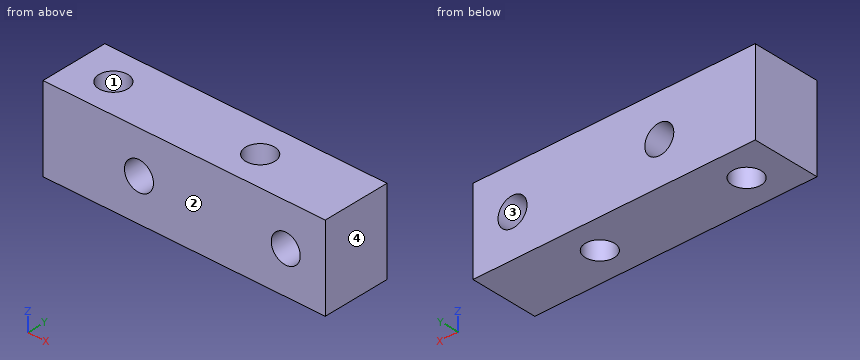
from build123d import *

# Parameters (mm, degrees)
SKETCH2_W               = 63.5
SKETCH2_H               = 19.05
BOSS_EXTRUDE1_DEPTH     = 15.24
F_1_4_CLEARANCE_HOLE2_D = 6.5278
F_1_4_CLEARANCE_HOLE3_D = 6.5278


with BuildPart() as part:
    # Sketch2 → Boss-Extrude1 (new body)
    with BuildSketch(Plane(origin=(0, 0, 0), x_dir=(1, 0, 0), z_dir=(0, 1, 0))):
        Rectangle(SKETCH2_W, SKETCH2_H)
    extrude(amount=-BOSS_EXTRUDE1_DEPTH)

    # 1/4 Clearance Hole2 (through all)
    with Locations(Plane.XY.offset(9.525)):
        with Locations((-22.86, -7.62), (10.16, -7.62)):
            Hole(F_1_4_CLEARANCE_HOLE2_D / 2)

    # 1/4 Clearance Hole3 (through all)
    with Locations(Plane(origin=(0, 0, 0), x_dir=(1, 0, 0), z_dir=(0, 1, 0))):
        with Locations((-10.16, 0), (22.86, 0)):
            Hole(F_1_4_CLEARANCE_HOLE3_D / 2)


solid = part.part
Here's how the part is built. I have some questions about the finished solid (model axes, mm). Face numbers are marked on the shaded views. Round coordinates to 2 decimals unless told otherwise and drop trailing zeros. Order: outer loops, then holes, each group sorted by start corner. A loop starts at its lowest first (then second) coordinate and runs counter-clockwise, first axis right, second up. Notation, with made-up numbers: M 88,-7 L 103,-7 A29 ccw 103,28 Z; hole C 8.5,3 d1. An arc over 180 degrees is marked long. One line per question, with ' | ' between items.
1) We'd pull the mould along X, two halves only. Please class the marked faces 1, 2, 3 and 4: released by +X, released by -X, zero draft, split by the parting line, or undercut.
Checked values:
face 1: undercut | face 2: zero draft | face 3: undercut | face 4: released by +X
2) Imagine slicing it at C-C, the plane x = -10.16. Write out the boundary of the cut face in (y, z) (3 decimals).
Checked values:
outline: M -15.24,-9.525 L 0,-9.525 L 0,-3.264 L -15.24,-3.264 Z; M -15.24,3.264 L 0,3.264 L 0,9.525 L -15.24,9.525 Z
3) Imagine slicing it at D-D, the plane z = -7. Write out the boundary of the cut face in (x, y), plus the area to 3 significant figures.
Checked values:
outline: M -31.75,-15.24 L 31.75,-15.24 L 31.75,0 L -31.75,0 Z; hole C -22.86,-7.62 d6.53; hole C 10.16,-7.62 d6.53 | area: 901 mm²
4) I need wall thicknesses on line 1 (Z direction, x = -10.16, y = -8) (3 decimals); line 2 (X direction, y = -7.5, z = 7); line 3 (X direction, y = -10, z = -2). Which ranges of each line are inside material? Lowest first, please.
Checked values:
line 1: z = -9.525 to -3.264, 3.264 to 9.525 | line 2: x = -31.75 to -26.12, -19.6 to 6.9, 13.42 to 31.75 | line 3: x = -31.75 to -25.09, -20.63 to -12.74, -7.58 to 7.93, 12.39 to 20.28, 25.44 to 31.75
5) Imagine slicing it at B-B, the plane z = 0. Write out the boundary of the cut face in (x, y).
Checked values:
outline: M -31.75,-15.24 L -13.42,-15.24 L -13.42,0 L -31.75,0 Z; M -6.9,-15.24 L 19.6,-15.24 L 19.6,0 L -6.9,0 Z; M 26.12,-15.24 L 31.75,-15.24 L 31.75,0 L 26.12,0 Z; hole C -22.86,-7.62 d6.53; hole C 10.16,-7.62 d6.53
6) Imagine slicing it at A-A, the plane y = -7.62. Write out the boundary of the cut face in (x, z) (3 decimals).
Checked values:
outline: M -31.75,-9.525 L -26.124,-9.525 L -26.124,9.525 L -31.75,9.525 Z; M -19.596,-9.525 L 6.896,-9.525 L 6.896,9.525 L -19.596,9.525 Z; M 13.424,-9.525 L 31.75,-9.525 L 31.75,9.525 L 13.424,9.525 Z; hole C -10.16,0 d6.528; hole C 22.86,0 d6.528
